```python
from build123d import *

# Parameters (mm, degrees)
F0_R     = 6.15
F1_DEPTH = 25
F2_R     = 3.15
F3_DEPTH = 4.5
F4_W     = 4
F4_H     = 43.2851596258
F5_DEPTH = 25.001
F6_R     = 8
F7_R     = 10
F8_R     = 3.15
F9_DEPTH = 1


with BuildPart() as f1:
    # F0 (on Top) → F1 (new body)
    with BuildSketch(Plane.XY):
        with BuildLine():
            Line((4.5, 7.3873202178), (-4.5, 7.3873202178))
            ThreePointArc((-4.5, 7.3873202178), (0, -8.65), (4.5, 7.3873202178))
        make_face()
        Circle(F0_R, mode=Mode.SUBTRACT)
    extrude(amount=F1_DEPTH)

    # F2 (on Right) → F3 (join, symmetric)
    with BuildSketch(Plane.YZ):
        with BuildLine():
            Line((34.739792331, 18.3796097241), (7.3873202178, 25))
            Line((7.3873202178, 25), (7.3873202178, 0))
            Line((7.3873202178, 0), (37.3873202178, 0))
            ThreePointArc((37.3873202178, 0), (42.2851596258, 10.0860082429), (34.739792331, 18.3796097241))
        make_face()
        with Locations((32.3873202178, 8.6602540378)):
            Circle(F2_R, mode=Mode.SUBTRACT)
    extrude(amount=F3_DEPTH, both=True)

    # F4 (on Top) → F5 (cut, through all)
    with BuildSketch(Plane.XY):
        with Locations((0, 21.6425798129)):
            Rectangle(F4_W, F4_H)
    extrude(amount=F5_DEPTH, mode=Mode.SUBTRACT)

    # F6
    f6_edges = [f1.edges().sort_by_distance(p)[0] for p in [
        (4.5, 7.38732, 12.5),
        (-4.5, 7.38732, 12.5),
    ]]
    fillet(f6_edges, radius=F6_R)

    # F7
    f7_edges = [f1.edges().sort_by_distance(p)[0] for p in [
        (-2, 5.815711, 12.5),
        (2, 5.815711, 12.5),
    ]]
    fillet(f7_edges, radius=F7_R)

    # F8 (on face) → F9 (cut)
    with BuildSketch(Plane(origin=(-4.5, 0, 0), x_dir=(0, -1, 0), z_dir=(-1, 0, 0))):
        Polygon((-37.5373202178, 11.6336079242), (-37.5373202178, 5.6869001515), (-32.3873202178, 2.7135462652), (-27.2373202178, 5.6869001515), (-27.2373202178, 11.6336079242), (-32.3873202178, 14.6069618105), align=None)
        with Locations((-32.3873202178, 8.6602540378)):
            Circle(F8_R, mode=Mode.SUBTRACT)
    extrude(amount=-F9_DEPTH, mode=Mode.SUBTRACT)


solid = f1.part
```
Here's how the part is built. I have some questions about the finished solid (model axes, mm). A direction names the side the tool comes from. Round coordinates to 2 decimals unless told otherwise and drop trailing zeros. Write each loop counter-clockwise with the first axis right and the second up, starting at its lowest first coordinate (ties: lowest second). Pieces come first, ordered by that corner, then holes.
Q1. Will these pins go through, and if not, where does the flat tip stop? P1, Ø3, axis at y = 32, z = 11.5, coming from the -X side; P2, Ø7.5, axis at y = 23, z = 15, coming from the +X side; P3, Ø2, axis at x = -1.5, z = 8, coming from the -Y side.
Q2. If we section it at D-D on z = 20.25: Write out the boundary of the cut face in (x, y), plus the area to 3 significant figures.
Q3. If we section it at C-C on z = 11: Write out the boundary of the cut face in (x, y).
Q4. Please list where these lines run through material, in increasing order: probe 1 along X at (y, z) = (13, 23.5); probe 2 along X at (y, z) = (0, 7.5); probe 3 along Y at (x, z) = (0, 18.25).
Q5. If we section it at A-A on x = -4: Write out the boundary of the cut face in (y, z).
Q6. If we section it at B-B on y = 0: Write out the boundary of the cut face in (x, z), plus the area to 3 significant figures.
Q7. If we mould it in two halves opening along Y, with no side actions, what happens to faces 6 (the flat face through (-3, 13, 0)), 7 (the cylindrical face through (2.646, 7.272, 12.325)), 8 (the cylindrical face through (-2.646, 7.272, 12.325)), 9 (the cylindrical face through (-3.232, 42.308, 9.921))? For each: +Y half, -Y half, draft (parallel to the pull), parting line (faces both ways), or undercut.
Q8. Which directions (+Z, -Z, +X, -X, +Y, -Y) give clear straight access to the entire face, cutting with the end or side of a thin tool? Please do faces 1 (the flat face through (4.5, 23, 10)), 2 (the flat face through (-2, 26, 9)), 3 (the cylindrical face through (-2.76, 30.066, 10.789)), 4 (the flat face through (-4.5, 23, 10)), 5 (the flat face through (-4.01, 29.85, 4.18)).
Answer below:
1. P1: stops at x = -3.5
1. P2: stops at x = 4.5
1. P3: stops at y = -8.64
2. outline: (-6.49, 5.71) arc R8.65 ccw (long way) to (6.49, 5.71) arc R8 cw to (4.5, 11) - (4.5, 27.01) - (2, 27.01) - (2, 10.81) arc R10 ccw to (4.57, 4.12) arc R6.15 cw (long way) to (-4.57, 4.12) arc R10 ccw to (-2, 10.81) - (-2, 27.01) - (-4.5, 27.01) - (-4.5, 11) arc R8 cw to start
2. area: 199 mm2
3. outline: (-6.49, 5.71) arc R8.65 ccw (long way) to (6.49, 5.71) arc R8 cw to (4.5, 11) - (4.5, 30.28) - (2, 30.28) - (2, 10.81) arc R10 ccw to (4.57, 4.12) arc R6.15 cw (long way) to (-4.57, 4.12) arc R10 ccw to (-2, 10.81) - (-2, 30.28) - (-3.5, 30.28) - (-3.5, 27.24) - (-4.5, 27.24) - (-4.5, 11) arc R8 cw to start; (-4.5, 37.54) - (-3.5, 37.54) - (-3.5, 34.5) - (-2, 34.5) - (-2, 42.11) - (-4.5, 42.11) - close; (2, 34.5) - (4.5, 34.5) - (4.5, 42.11) - (2, 42.11) - close
4. probe 1: x = -4.5 to -2, 2 to 4.5
4. probe 2: x = -8.65 to -6.15, 6.15 to 8.65
4. probe 3: y = -8.65 to -6.15
5. outline: (-7.67, 0) - (-4.67, 0) - (-4.67, 25) - (-7.67, 25) - close; (4.81, 0) - (37.39, 0) arc R10 ccw to (34.74, 18.38) - (7.39, 25) - (4.81, 25) - close; hole (27.24, 5.69) - (32.39, 2.71) - (37.54, 5.69) - (37.54, 11.63) - (32.39, 14.61) - (27.24, 11.63) - close
6. outline: (-8.65, 0) - (-6.15, 0) - (-6.15, 25) - (-8.65, 25) - close; (6.15, 0) - (8.65, 0) - (8.65, 25) - (6.15, 25) - close
6. area: 125 mm2
7. face 6: draft
7. face 7: undercut
7. face 8: undercut
7. face 9: +Y half
8. face 1: +Z, -Z, +X, +Y
8. face 2: +Z, -Z, +Y
8. face 3: +X, -X
8. face 4: +Z, -Z, -X, +Y
8. face 5: -X
